Build history of the part. All positions in model axes, mm. Coordinates: 2 decimals unless noted, no trailing zeros. Write each loop counter-clockwise with the first axis right and the second up, starting at its lowest first coordinate (ties: lowest second). Pieces come first, ordered by that corner, then holes. Notation, with made-up numbers: (-4.5, 36.5) -> (38.5, 36.5) arc R20 ccw to (38.5, 53.5) -> close; hole circle Ø3 at (-37, 86.25). An arc over 180 degrees is marked (long way). Write each question's results on one line, items separated by ' | '. Start each with the question number.
Q1. Saw through at B-B on y = -117.5. Give the cut face in (x, z), and give its area (3 significant figures).
Q2. Drill centre lines: line 1 (X direction, y = -112.5, z = -56); line 2 (X direction, y = -44, z = -39.5). Where is each one in solid material? Low to high.
Q3. Saw through at C-C on x = 1. Give the cut face in (y, z), and give its area (3 significant figures).
Q4. Drop flat-ended pins along their axis: pin 1 Ø1.5 at (y, z) = (-122, -19.5) entering from +X; pin 2 Ø12 at (y, z) = (-62.5, -121) entering from -X; pin 3 Ø5 at (y, z) = (-89.5, -43) entering from +X. Give the stop position or say it passes through.
Q5. Two-plate mould, pull along Y, no slides. Class faces 1 (the face through (23.396, -61.895, -116.85)), 2 (the face through (-5, -135, -110.465)), 3 (the face through (-6.667, -134.712, -141.784)): released by +Y, released by -Y, zero draft, split by the parting line, or undercut.
Autodesk Inventor part; units mm, degrees
ref_plane "作業平面2" through (-8.85, -128.1353, -159.8711) normal (0, 0.3826834, -0.9238795) x (0, 0.9238795, 0.3826834)
ref_plane "作業平面4" through (-7.8771, -140.7638, -110.4647) normal (0, 0, 1) x (1, 0, 0)
ref_plane "YZ Plane" through (0, 0, 0) normal (1, 0, 0) x (0, 1, 0)
ref_plane "作業平面1" through (14.25, -85.0419, 0) normal (0, 0, -1) x (0, 1, 0)
sketch "スケッチ1" plane through (14.25, -85.0419, 0) normal (0, 0, -1) x (0, 1, 0)
  line L0 (-46.6818, -19.75) -> (47.5988, 17.4243)
  line L1 (47.5988, 17.4243) -> (46.6818, 19.75)
  line L2 (46.6818, 19.75) -> (-47.5988, -17.4243)
  line L3 (-47.5988, -17.4243) -> (-46.6818, -19.75)
  point P0 (85.0419, -14.25)
ref_plane "作業平面2" through (-8.85, -128.1353, -159.8711) normal (0, 0.3826834, -0.9238795) x (0, 0.9238795, 0.3826834)
extrude "押し出し1" add sketch "スケッチ1" along normal up to surface surface through (-8.85, -128.1353, -159.8711) normal (0, 0.3826834, -0.9238795)
sketch "スケッチ2" plane through (-3.1743, -132.6408, 0) normal (0.930296, -0.3668097, 0) x (0, 0, -1)
  line L0 (0, 30.3562) -> (10, 30.3562)
  line L1 (0, 91.3953) -> (0, 30.3562)
  line L2 (10, 91.3953) -> (0, 91.3953)
  line L3 (10, 30.3562) -> (10, 91.3953)
  line L4 (110.4647, 30.3562) -> (120.4647, 30.3562)
  line L5 (110.4647, 91.3953) -> (110.4647, 30.3562)
  line L6 (120.4647, 91.3953) -> (110.4647, 91.3953)
  line L7 (120.4647, 30.3562) -> (120.4647, 91.3953)
  line L8 (110.4647, 30.3562) -> (120.4647, 30.3562)
  line L9 (110.4647, 91.3953) -> (110.4647, 30.3562)
  line L10 (120.4647, 91.3953) -> (110.4647, 91.3953)
  line L11 (120.4647, 30.3562) -> (120.4647, 91.3953)
  line L12 (0, 91.3953) -> (10, 91.3953)
  line L13 (10, 91.3953) -> (10, 60.8757)
  line L14 (10, 60.8757) -> (0, 60.8757)
  line L15 (0, 60.8757) -> (0, 91.3953)
  line L16 (10, 60.8757) -> (0, 60.8757)
  line L17 (0, 60.8757) -> (0, 30.3562)
  line L18 (0, 30.3562) -> (10, 30.3562)
  line L19 (10, 30.3562) -> (10, 60.8757)
  line L20 (110.4647, 91.3953) -> (120.4647, 91.3953)
  line L21 (120.4647, 91.3953) -> (120.4647, 60.8757)
  line L22 (120.4647, 60.8757) -> (110.4647, 60.8757)
  line L23 (110.4647, 60.8757) -> (110.4647, 91.3953)
  line L24 (120.4647, 60.8757) -> (110.4647, 60.8757)
  line L25 (110.4647, 60.8757) -> (110.4647, 30.3562)
  line L26 (110.4647, 30.3562) -> (120.4647, 30.3562)
  line L27 (120.4647, 30.3562) -> (120.4647, 60.8757)
  circle A0 centre (5, 45.616) radius 1.5
  circle A1 centre (5, 76.1355) radius 1.5
  circle A2 centre (115.4647, 76.1355) radius 1.5
  circle A3 centre (115.4647, 45.616) radius 1.5
  circle A4 centre (115.4647, 76.1355) radius 1.5
  circle A5 centre (115.4647, 45.616) radius 1.5
  circle A6 centre (5, 76.1355) radius 1.5
  circle A7 centre (5, 45.616) radius 1.5
  circle A8 centre (115.4647, 76.1355) radius 1.5
  circle A9 centre (115.4647, 45.616) radius 1.5
  point P0 (0, 124.5595)
  dimension "d2" = 3
  dimension "d3" = 3
  dimension "d4" = 3
  dimension "d5" = 3
extrude "押し出し2" cut sketch "スケッチ2" against normal blind 2.5 contours A0 | A1 | A2 | A3
ref_plane "作業平面3" through (13.1229, -86.9061, -10) normal (0, 0, -1) x (0, 1, 0)
sketch "スケッチ3" plane through (13.1229, -86.9061, -10) normal (0, 0, -1) x (0, 1, 0)
  line L0 (-44.8176, -18.6229) -> (-45.7346, -16.2971)
  line L1 (-50.8753, -21) -> (-51.7923, -18.6743)
  line L2 (-53.8577, -21) -> (53.8577, -21)
  line L3 (-45.423, -16.1743) -> (-53.8577, -19.5)
  line L4 (-51.7923, -18.6743) -> (-50.8753, -21)
  line L5 (-50.8753, -21) -> (-44.8215, -18.613)
  line L6 (-44.8215, -18.613) -> (-45.7385, -16.2873)
  line L7 (-45.7385, -16.2873) -> (-51.7923, -18.6743)
  point P0 (86.9061, -13.1229)
  point P1 (-51.7884, -18.6841)
ref_plane "作業平面4" through (-7.8771, -140.7638, -110.4647) normal (0, 0, 1) x (1, 0, 0)
extrude "押し出し3" add sketch "スケッチ3" along normal up to surface (100.4647 mm away) contours L5 L1 L3 L0
ref_plane "作業平面5" through (13.1229, -86.9061, -120.4647) normal (0, 0, -1) x (0, 1, 0)
sketch "スケッチ4" plane through (13.1229, -86.9061, -120.4647) normal (0, 0, -1) x (0, 1, 0)
  line L0 (-44.8176, -18.6229) -> (-45.7346, -16.2971)
  line L1 (-50.8753, -21) -> (-51.7923, -18.6743)
  line L2 (49.4342, 18.5514) -> (-50.8753, -21)
  line L3 (-51.7923, -18.6743) -> (48.5172, 20.8771)
  line L4 (-45.7346, -16.2971) -> (-44.8176, -18.6229)
  line L5 (-44.8176, -18.6229) -> (-50.8714, -21.0098)
  line L6 (-50.8714, -21.0098) -> (-51.7884, -18.6841)
  line L7 (-51.7884, -18.6841) -> (-45.7346, -16.2971)
  point P0 (86.9061, -13.1229)
  point P1 (-51.7884, -18.6841)
  point P2 (-44.8215, -18.613)
extrude "押し出し4" add sketch "スケッチ4" along normal up to surface contours L2 L1 L7 L0 surface through (14.25, -85.0419, -142.0212) normal (0, 0.3826834, -0.9238795)
sketch "スケッチ7" plane through (34, -38.3601, 0) normal (0.930296, -0.3668097, 0) x (0, 0, -1)
  circle A0 centre (5, -55.7288) radius 1.5
  circle A1 centre (115.4647, -55.7288) radius 1.5
  circle A2 centre (5, -25.2093) radius 1.5
  circle A3 centre (115.4647, -25.2093) radius 1.5
  line L0 (164.2448, -107.8521) -> (122.685, 0)
  line L1 (0, 0) -> (122.685, 0)
  line L2 (0, 0) -> (0, -101.3448)
  line L3 (0, -101.3448) -> (10, -101.3448)
  line L4 (10, -101.3448) -> (10, -107.8521)
  line L5 (10, -107.8521) -> (110.4647, -107.8521)
  line L6 (110.4647, -101.3448) -> (110.4647, -107.8521)
  line L7 (110.4647, -101.3448) -> (120.4647, -101.3448)
  line L8 (120.4647, -101.3448) -> (120.4647, -107.8521)
  line L9 (120.4647, -107.8521) -> (164.2448, -107.8521)
  line L10 (122.1491, 0) -> (163.709, -107.8521)
  line L11 (164.2448, -107.8521) -> (122.685, 0)
  point P0 (0, 23.2147)
  dimension "d13" = 0.5
extrude "押し出し5" cut sketch "スケッチ7" against normal blind 2.5 contours L9 L10 L1 L0
properties part number "lefft_wall" material "木材 (カエデ材)"
Returned:
1) outline: (0.11, -155.31) -> (2.8, -154.93) -> (2.8, 0) -> (0.11, 0) -> close | area: 417 mm2
2) line 1: x = 2.08 to 4.77 | line 2: x = 29.09 to 31.78
3) outline: (-122.05, -156.82) -> (-115.24, -154.37) -> (-115.24, 0) -> (-122.05, 0) -> close | area: 1,060 mm2
4) pin 1: stops at x = 1.32 | pin 2: stops at x = 19.43 | pin 3: stops at x = 14.82
5) face 1: undercut | face 2: zero draft | face 3: released by +Y
